Autodesk Inventor part; units mm, degrees
ref_plane "YZ Plane" through (0, 0, 0) normal (1, 0, 0) x (0, 1, 0)
ref_plane "XZ Plane" through (0, 0, 0) normal (0, 1, 0) x (-1, 0, 0)
ref_plane "XY Plane" through (0, 0, 0) normal (0, 0, 1) x (1, 0, 0)
sketch "Sketch1" plane through (0, 0, 0) normal (0, 0, 1) x (1, 0, 0)
  line L0 (-40, 40) -> (40, 40)
  line L1 (40, 40) -> (40, -40)
  line L2 (40, -40) -> (-40, -40)
  line L3 (-40, -40) -> (-40, 40)
  point P0 (0, 0)
  dimension "d0" = 80
  dimension "d1" = 80
  dimension "d19" = 40
  dimension "d20" = 40
extrude "Extrusion1" add sketch "Sketch1" along normal blind 0.3
sketch "Sketch2" plane through (0, 0, 0.3) normal (0, 0, 1) x (1, 0, 0)
  line L0 (40, 40) -> (-40, 40)
  line L1 (-40, 40) -> (-40, -40)
  line L2 (-40, -40) -> (40, -40)
  line L3 (40, -40) -> (40, 40)
  line L4 (-41, 41) -> (41, 41)
  line L5 (41, 41) -> (41, -41)
  line L6 (41, -41) -> (-41, -41)
  line L7 (-41, -41) -> (-41, 41)
  point P0 (0, 0)
  dimension "d4" = 1
extrude "Extrusion2" add sketch "Sketch2" against normal blind 5
fillet "Fillet1" radius 2 8 edges at (40, 40, -2.35) (-40, 40, -2.35) (40, -40, -2.35) (-40, -40, -2.35) (41, 41, -2.2) (-41, 41, -2.2) (-41, -41, -2.2) (41, -41, -2.2)
sketch "Sketch3" plane through (40, -38, 0) normal (-1, 0, 0) x (0, 0, 1)
  line L0 (-4.7, 77) -> (-4.7, -1)
  line L1 (-4.7, 48) -> (-1.7, 48)
  line L2 (-1.7, 48) -> (-1.7, 28)
  line L3 (-1.7, 28) -> (-4.7, 28)
  line L4 (-4.7, 28) -> (-4.7, 48)
  line L5 (0, 78) -> (-4.7, 78)
  point P0 (0, 38)
  dimension "d13" = 3
  dimension "d14" = 20
  dimension "d15" = 30
extrude "Extrusion3" add sketch "Sketch3" along normal blind 1.5
chamfer "Chamfer1" distance 1 angle 45 1 edges at (38.5, 0, -1.7)
chamfer "Chamfer2" distance 1 angle 45 1 edges at (38.5, 0, -4.7)
pattern_circular "Circular Pattern1" count 3 over 180 about axis through (0, 0, -10) along (0, 0, 1) of "Extrusion3", "Chamfer2", "Chamfer1"
sketch "Sketch4" plane through (0, 0, -4.7) normal (0, 0, -1) x (-1, 0, 0)
  line L0 (38, -40) -> (-38, -40)
  arc A0 (-0.8, -40) -> (0.8, -40) centre (0, -40) ccw
  point P0 (0, 0)
  dimension "d24" = 0.8
extrude "Extrusion4" cut sketch "Sketch4" against normal up to surface (4.7 mm away)
properties part number "Cap plate"
Source: CAD feature listing. Evaluate the final solid. Frame: model axes, mm. A direction names the side the tool comes from. Coordinates: 2 decimals unless noted, no trailing zeros. Order: outer loops, then holes, each group sorted by start corner. A loop starts at its lowest first (then second) coordinate and runs counter-clockwise, first axis right, second up. Notation, with made-up numbers: (88, -23) - (103, -23) arc R38 ccw to (103, 15) - close; hole circle Ø7 at (25.5, -29.75). An arc over 180 degrees is marked (long way). One line per item, written item: value.
1) Contact query for flat-ended pins moving along their axis: pin 1 (0.8 mm diameter, centred on x = -39.5, z = -3.5, fed in from +Y); pin 2 (4 mm diameter, centred on x = 28.5, y = 31, fed in from -Z). Output: stop coordinate, or through.
Computed values:
pin 1: stops at y = 41
pin 2: stops at z = 0
2) Mould query, pull axis Y, two halves, no side actions, for faces 4 (the face through (-1, 1, 0.3)), 5 (the face through (19, -40, -2)), 6 (the face through (40.43, -40.4, -2.24)), 7 (the face through (39.4, 39.43, -2.38)). Classes: released by +Y, released by -Y, zero draft, split by the parting line, or undercut.
Computed values:
face 4: zero draft
face 5: undercut
face 6: released by -Y
face 7: undercut
3) Cut plane A-A on x = -26. Output: boundary loops of the cut face in (y, z), plus the area to 3 significant figures.
Computed values:
outline: (-41, -4.7) - (-40, -4.7) - (-40, 0) - (40, 0) - (40, -4.7) - (41, -4.7) - (41, 0.3) - (-41, 0.3) - close
area: 34.0 mm^2
4) Ray query, line 1 (Y direction, x = -32, z = -0.5); line 2 (Y direction, x = 5, z = -2.95). Return the intervals inside material, ascending. Write a range as [from, to].
Computed values:
line 1: y = [-41, -40], [40, 41]
line 2: y = [-41, -40], [38.5, 41]
5) Reachability of faces 1 (the face through (-39.43, 39.4, -2.38)), 2 (the face through (-40, 1, -1)), 3 (the face through (40.4, 40.43, -2.24)) from +Z, -Z, +X, -X, +Y, -Y: full face, straight path, thin tool, end or side. Return the list, or none.
Computed values:
face 1: -Z
face 2: none
face 3: +Z, -Z, +X, +Y
6) Cut plane C-C on y = 4. Output: boundary loops of the cut face in (x, z).
Computed values:
outline: (-41, -4.7) - (-39.5, -4.7) - (-38.5, -3.7) - (-38.5, -2.7) - (-39.5, -1.7) - (-40, -1.7) - (-40, 0) - (40, 0) - (40, -1.7) - (39.5, -1.7) - (38.5, -2.7) - (38.5, -3.7) - (39.5, -4.7) - (41, -4.7) - (41, 0.3) - (-41, 0.3) - close
